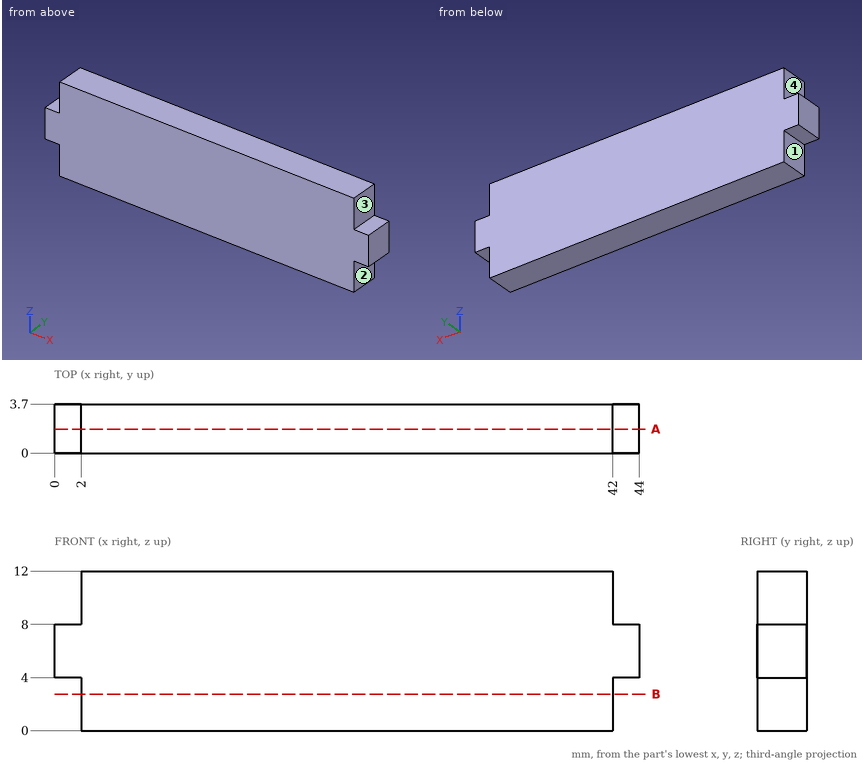
Input: dimensioned drawing with shaded views. Units: mm. Origin: part minimum x, y, z. A direction names the side the tool comes from. Round coordinates to 2 decimals unless told otherwise and drop trailing zeros. Loops run counter-clockwise (first coordinate to the right, second up) from the corner with the lowest first, then second, coordinate; pieces in that order, holes last. Notation, with made-up numbers: (50.25, 27.25) -> (58.25, 27.25) arc R15 cw to (58.25, 35.25) -> close; hole circle Ø1 at (21.25, 42). An arc over 180 degrees is marked (long way). Use one line per item in the form item = value. Start each with the question number.
1) Section B-B on z = 2.75. Output: boundary loops of the cut face in (x, y), then the cut area to 3 significant figures.
2) Line query: L1, parallel to X at y = 0.7, z = 10.75. Output: solid intervals per line, ascending.
3) First-contact query: P1, Ø1, axis at x = 43, y = 2, coming from the +Z side; P2, Ø0.6, axis at x = 1, y = 1, coming from the -Z side; P3, Ø1.1, axis at y = 1, z = 1, coming from the -X side. Flat tips, straight axial feed; report the tip coordinate or a pass-through.
4) Section A-A on y = 1.8. Output: boundary loops of the cut face in (x, z).
5) Access query for the marked faces 1, 2, 3 and 4. Directions: +Z, -Z, +X, -X, +Y, -Y. A direction counts if a zero-diameter tool reaches every point of the face in a straight line with its end or side. Return the directions, or none.
Response:
q1.outline = (2, 0) -> (42, 0) -> (42, 3.7) -> (2, 3.7) -> close
q1.area = 148 mm^2
q2.L1 = 2 to 42
q3.P1 = 8
q3.P2 = 4
q3.P3 = 2
q4.outline = (0, 4) -> (2, 4) -> (2, 0) -> (42, 0) -> (42, 4) -> (44, 4) -> (44, 8) -> (42, 8) -> (42, 12) -> (2, 12) -> (2, 8) -> (0, 8) -> close
q5.face_1 = -Z, -X, +Y, -Y
q5.face_2 = -Z, +X, +Y, -Y
q5.face_3 = +Z, +X, +Y, -Y
q5.face_4 = +Z, -X, +Y, -Y
